from build123d import *

# Parameters (mm, degrees)
SKETCH1_W           = 6.35
SKETCH1_H           = 6.35
BOSS_EXTRUDE1_DEPTH = 8.89
FILLET1_R           = 0.635


with BuildPart() as part:
    # Sketch1 → Boss-Extrude1 (new body)
    with BuildSketch(Plane.XY):
        Polygon((7.332348419, 0), (3.666174209, 6.35), (-3.666174209, 6.35), (-7.332348419, 0), (-3.666174209, -6.35), (3.666174209, -6.35), align=None)
        Rectangle(SKETCH1_W, SKETCH1_H, mode=Mode.SUBTRACT)
    extrude(amount=BOSS_EXTRUDE1_DEPTH)

    # Fillet1
    fillet1_edges = [part.edges().sort_by_distance(p)[0] for p in [
        (0, 6.35, 8.89),
        (-5.499261314, 3.175, 8.89),
        (3.175, 0, 0),
        (0, 3.175, 0),
        (-3.175, 0, 0),
        (-5.499261314, -3.175, 8.89),
        (0, -3.175, 0),
        (3.175, 0, 8.89),
        (0, 3.175, 8.89),
        (-3.175, 0, 8.89),
        (0, -3.175, 8.89),
        (0, -6.35, 8.89),
        (5.499261314, -3.175, 8.89),
        (0, -6.35, 0),
        (-5.499261314, -3.175, 0),
        (-5.499261314, 3.175, 0),
        (0, 6.35, 0),
        (5.499261314, 3.175, 0),
        (5.499261314, -3.175, 0),
        (5.499261314, 3.175, 8.89),
    ]]
    fillet(fillet1_edges, radius=FILLET1_R)


solid = part.part
The model under review builds one solid part; all positions refer to its coordinate system, in mm. A direction names the side the tool comes from. Coordinates: 2 decimals unless noted, no trailing zeros. Loops run counter-clockwise (first coordinate to the right, second up) from the corner with the lowest first, then second, coordinate; pieces in that order, holes last. Notation, with made-up numbers: M 71,52.25 L 101,52.25 A19 cw 101,85.25 Z; hole C 49,20.5 d10. An arc over 180 degrees is marked long. Put each result on its own line as item: value. Start each with the question number.
Q1. The part is to be moulded in two halves that separate along X. For faces 1 (the cylindrical face through (5.4, -3, 0.2)), 2 (the flat face through (-5.525, -3.131, 4.392)), 3 (the flat face through (0, -3.175, 4)), say which applies: +X half, -X half, draft (parallel to the pull), parting line (faces both ways), or undercut.
Q2. For faces 4 (the flat face through (0, 3.175, 4)), 5 (the cylindrical face through (-5.317, -3.129, 0.191)), list the 3-axis set-ups (+Z, -Z, +X, -X, +Y, -Y) from which the entire face can be reached by the end or side of a thin tool; tool diameter is ignored.
Q3. Wall thickness on line 1 (Y direction, x = 1, z = 2.25) (3 decimals); line 2 (Z direction, x = 3.75, y = 3.5); line 3 (X direction, y = 0.5, z = 1.5) (3 decimals): over which ranges is each line inside the solid? List them lowest first.
Q4. Add section A-A (z = 3.5). Write out the cut boundary in (x, y) (3 decimals).
Q5. Clearance check with flat-ended pins moving along their axes: pin 1 (4 mm diameter, centred on y = 4, z = 4.5, fed in from +X); pin 2 (1.5 mm diameter, centred on y = -2.5, z = 2.5, fed in from +X); pin 3 (1 mm diameter, centred on y = 1, z = 2, fed in from +X). State where each tip first meets the part, or that it passes through.
Q6. Add section B-B (x = 3). Write out the cut boundary in (y, z) (3 decimals).
Answers:
1. face 1: +X half
1. face 2: -X half
1. face 3: undercut
2. face 4: +Z, -Z
2. face 5: -Z, -X, -Y
3. line 1: y = -6.35 to -3.175, 3.175 to 6.35
3. line 2: z = 0 to 8.89
3. line 3: x = -7.044 to -3.175, 3.175 to 7.044
4. outline: M -7.332,0 L -3.666,-6.35 L 3.666,-6.35 L 7.332,0 L 3.666,6.35 L -3.666,6.35 Z; hole M -3.175,-3.175 L 3.175,-3.175 L 3.175,3.175 L -3.175,3.175 Z
5. pin 1: stops at x = 6.18
5. pin 2: stops at x = 6.32
5. pin 3: stops at x = 7.04
6. outline: M -6.35,0.635 A0.635 ccw -5.715,0 L -3.81,0 A0.635 ccw -3.175,0.635 L -3.175,8.255 A0.635 ccw -3.81,8.89 L -5.715,8.89 A0.635 ccw -6.35,8.255 Z; M 3.175,0.635 A0.635 ccw 3.81,0 L 5.715,0 A0.635 ccw 6.35,0.635 L 6.35,8.255 A0.635 ccw 5.715,8.89 L 3.81,8.89 A0.635 ccw 3.175,8.255 Z
